Read the model definition and answer for the solid it produces. Units are mm, in the model's axes. A direction names the side the tool comes from. Coordinates: 2 decimals unless noted, no trailing zeros. Order: outer loops, then holes, each group sorted by start corner. A loop starts at its lowest first (then second) coordinate and runs counter-clockwise, first axis right, second up. Notation, with made-up numbers: (29.25, -32.75) - (56.25, -32.75) arc R22 ccw to (56.25, -6.75) - close; hole circle Ø10 at (62.25, -35.75). An arc over 180 degrees is marked (long way). Answer as a JSON object with one key per item and string values. Group by question number.
from build123d import *

# Parameters (mm, degrees)
ESQUISSE1_R                  = 125
ESQUISSE1_R_2                = 12.6
BOSS_EXTRU_1_DEPTH           = 6
ESQUISSE2_W                  = 10
ESQUISSE2_H                  = 25
ENL_V_MAT_EXTRU_1_DEPTH      = 7
R_P_TITION_CIRCULAIRE1_COUNT = 8


with BuildPart() as part:
    # Esquisse1 → Boss.-Extru.1 (new body)
    with BuildSketch(Plane.XY):
        Circle(ESQUISSE1_R)
        Circle(ESQUISSE1_R_2, mode=Mode.SUBTRACT)
    extrude(amount=BOSS_EXTRU_1_DEPTH)

    # Esquisse2 → Enlèv. mat.-Extru.1 (cut, through all)
    with BuildSketch(Plane(origin=(0, 0, 0), x_dir=(-1, 0, 0), z_dir=(0, 0, -1))):
        with Locations((0, 112.5)):
            Rectangle(ESQUISSE2_W, ESQUISSE2_H)
    enl_v_mat_extru_1 = extrude(amount=-ENL_V_MAT_EXTRU_1_DEPTH, mode=Mode.SUBTRACT)

    # Répétition circulaire1: Enlèv. mat.-Extru.1 ×8 about axis
    r_p_tition_circulaire1_axis = Axis((0, 0, 0), (0, 0, 1))
    for i in range(1, R_P_TITION_CIRCULAIRE1_COUNT):
        add(enl_v_mat_extru_1.rotate(r_p_tition_circulaire1_axis, i * 360 / R_P_TITION_CIRCULAIRE1_COUNT), mode=Mode.SUBTRACT)


solid = part.part
1. A cutting plane is placed at D-D on x = 51.5. Write down the section's boundary in (y, z), and give its area (3 significant figures).
2. For faces 5 (the flat face through (-112, -5, 3)), 6 (the flat face through (70.66, -70.76, 2.96)), 7 (the flat face through (-5, -112, 3)), 8 (the cylindrical face through (47.26, -115.72, 2.96)), determine the directions among +Z, -Z, +X, -X, +Y, -Y from which every point of the face is accessible in a straight line to the end or side of a thin tool.
3. For a pull along X with two mould halves and no side action, classify faces 1 (the cylindrical face through (-115.72, -47.26, 2.96)), 2 (the flat face through (-70.76, -70.66, 2.96)), 3 (the flat face through (-112, 5, 3)), 4 (the flat face through (-82.93, 75.86, 2.96)) as pulls with the +X half, pulls with the -X half, needs draft (parallel to the pull), parting line crosses it, or undercut.
4. Given pin 1 (3 mm diameter, centred on y = 2.5, z = 2, fed in from -X); pin 2 (3 mm diameter, centred on x = -110, z = 3.5, fed in from +Y); pin 3 (3 mm diameter, centred on x = -1.5, z = 2, fed in from +Y), each flat-ended and moving along its own axis, determine where each tip first touches the part or whether it passes through.
5. A cutting plane is placed at A-A on x = 0. Write down the section's boundary in (y, z).
6. Straight lines are drawn through the part: L1, parallel to Y at x = 0, z = 3.35; L2, parallel to X at y = -77.5, z = 1.45; L3, parallel to X at y = -78, z = 1.3. For each, find the intervals that lie inside material, in ascending order.
Derived:
{
 "1": {"outline": "(-113.9, 0) - (113.9, 0) - (113.9, 6) - (-113.9, 6) - close", "area": "1,370 mm2"},
 "2": {"face 5": "+Z, -Z, -X", "face 6": "+Z, -Z", "face 7": "+Z, -Z, -Y", "face 8": "+Z, -Z, +X, -Y"},
 "3": {"face 1": "pulls with the -X half", "face 2": "undercut", "face 3": "needs draft", "face 4": "undercut"},
 "4": {"pin 1": "stops at x = -100", "pin 2": "stops at y = 62.07", "pin 3": "stops at y = 100"},
 "5": {"outline": "(-100, 0) - (-12.6, 0) - (-12.6, 6) - (-100, 6) - close; (12.6, 0) - (100, 0) - (100, 6) - (12.6, 6) - close"},
 "6": {"L1": "y = -100 to -12.6, 12.6 to 100", "L2": "x = -98.08 to -84.57, -70.43 to 70.43, 84.57 to 98.08", "L3": "x = -97.68 to -85.07, -70.93 to 70.93, 85.07 to 97.68"}
}
